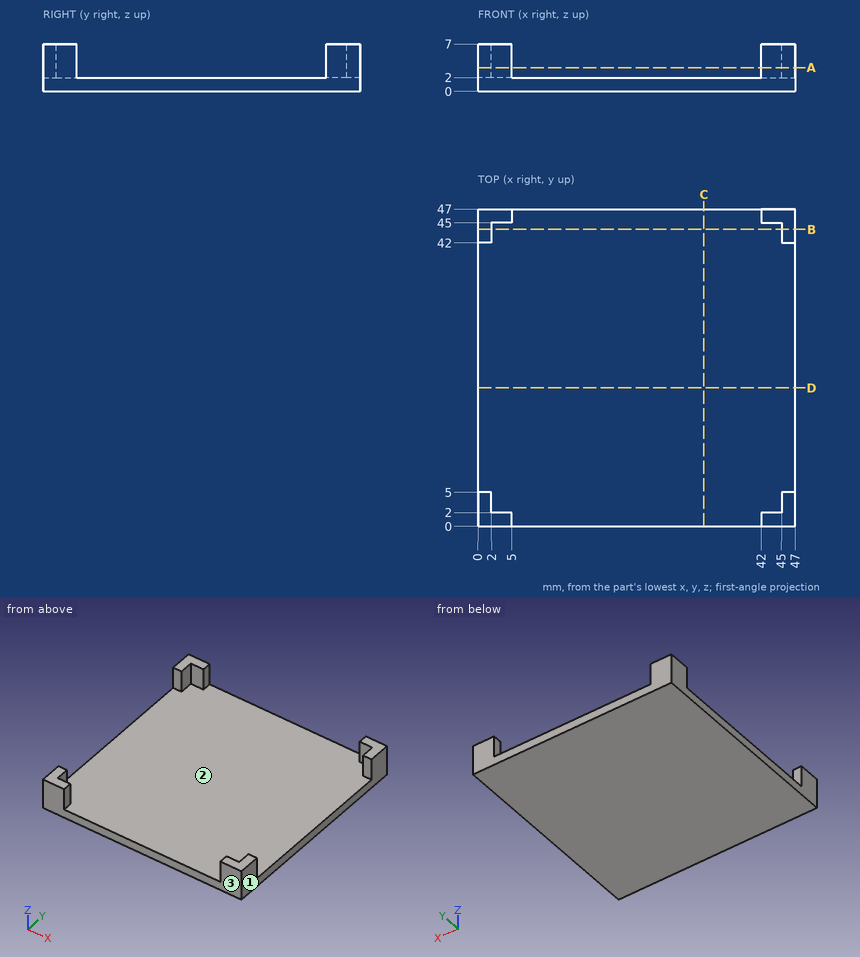
The figure shows three views and two pictorial views of one solid part (mm, origin at its lowest corner). Answer the questions. Round coordinates to 2 decimals unless told otherwise and drop trailing zeros. Order: outer loops, then holes, each group sorted by start corner. A loop starts at its lowest first (then second) coordinate and runs counter-clockwise, first axis right, second up. Notation, with made-up numbers: (65, 8) - (92, 8) arc R18 ccw to (92, 25) - close; hole circle Ø6 at (35, 21.25). An arc over 180 degrees is marked (long way). Write item = value, one per line. Start each with the question number.
1) Straight lines are drawn through the part: L1, parallel to Y at x = 4.5, z = 5.5; L2, parallel to Z at x = 43.5, y = 23. For each, find the intervals that lie inside material, in ascending order.
2) Section C-C, the plane x = 33.5 is taken. Write down the section's boundary in (y, z).
3) Section A-A, the plane z = 3.5 is taken. Write down the section's boundary in (x, y), plus the area to 3 significant figures.
4) Section B-B, the plane y = 44 is taken. Write down the section's boundary in (x, z), plus the area to 3 significant figures.
5) For a pull along Y with two mould halves and no side action, classify the marked faces 1, 2 and 3 as released by +Y, released by -Y, zero draft, split by the parting line, or undercut.
6) Given pin 1 (5 mm diameter, centred on x = 31, y = 27, fed in from +Z), flat-ended and moving along its own axis, determine where the tip first touches the part or whether it passes through.
Results list:
q1.L1 = 0 to 2, 45 to 47
q1.L2 = 0 to 2
q2.outline = (0, 0) - (47, 0) - (47, 2) - (0, 2) - close
q3.outline = (0, 0) - (5, 0) - (5, 2) - (2, 2) - (2, 5) - (0, 5) - close; (0, 42) - (2, 42) - (2, 45) - (5, 45) - (5, 47) - (0, 47) - close; (42, 0) - (47, 0) - (47, 5) - (45, 5) - (45, 2) - (42, 2) - close; (42, 45) - (45, 45) - (45, 42) - (47, 42) - (47, 47) - (42, 47) - close
q3.area = 64.0 mm^2
q4.outline = (0, 0) - (47, 0) - (47, 7) - (45, 7) - (45, 2) - (2, 2) - (2, 7) - (0, 7) - close
q4.area = 114 mm^2
q5.face_1 = zero draft
q5.face_2 = undercut
q5.face_3 = released by -Y
q6.pin_1 = 2
